Autodesk Inventor part; units mm, degrees
ref_plane "YZ Plane" through (0, 0, 0) normal (1, 0, 0) x (0, 1, 0)
ref_plane "XZ Plane" through (0, 0, 0) normal (0, 1, 0) x (-1, 0, 0)
ref_plane "XY Plane" through (0, 0, 0) normal (0, 0, 1) x (1, 0, 0)
sketch "Эскиз1" plane through (0, 0, 0) normal (0, 0, 1) x (1, 0, 0)
  line L0 (-74.5, -35) -> (74.5, -35)
  line L1 (74.5, -35) -> (74.5, 35)
  line L2 (74.5, 35) -> (-74.5, 35)
  line L3 (-74.5, 35) -> (-74.5, -35)
  line L4 (-74.5, -35) -> (74.5, 35) construction
  line L5 (74.5, -35) -> (-74.5, 35) construction
  point P0 (0, 0)
  dimension "d0" = 149
  dimension "d1" = 70
extrude "Выдавливание1" add sketch "Эскиз1" along normal blind 3
sketch "Эскиз2" plane through (0, 0, 3) normal (0, 0, 1) x (1, 0, 0)
  line L0 (74.5, -35) -> (74.5, 35)
  line L1 (74.5, 25) -> (71.5, 25)
  line L2 (71.5, 25) -> (71.5, 15)
  line L3 (71.5, 15) -> (74.5, 15)
  line L4 (74.5, 15) -> (74.5, 25)
  line L5 (74.5, 35) -> (-74.5, 35)
  point P0 (0, 0)
  dimension "d4" = 3
  dimension "d5" = 10
  dimension "d6" = 10
extrude "Выдавливание2" cut sketch "Эскиз2" against normal blind 3
pattern_linear "Прямоуг.массив1" count 3 spacing 20 along (0, -1, 0) of "Выдавливание2"
mirror "Зеркальное отражение1" about plane through (0, 0, 0) normal (1, 0, 0) of "Выдавливание2", "Прямоуг.массив1"
sketch "Эскиз3" plane through (0, 0, 3) normal (0, 0, 1) x (1, 0, 0)
  line L0 (-74.5, -35) -> (74.5, -35)
  line L1 (-50, -35) -> (50, -35)
  line L2 (50, -35) -> (50, -38)
  line L3 (50, -38) -> (-50, -38)
  line L4 (-50, -38) -> (-50, -35)
  line L5 (0, 0) -> (0, -8.2609)
  line L6 (-74.5, -25) -> (-74.5, -35)
  dimension "d12" = 3
  dimension "d13" = 24.5
extrude "Выдавливание3" add sketch "Эскиз3" against normal blind 3
sketch "Эскиз4" plane through (0, 0, 3) normal (0, 0, 1) x (1, 0, 0)
  line L0 (74.5, 35) -> (-74.5, 35)
  line L1 (-74.5, 35) -> (-64.5, 35)
  line L2 (-64.5, 35) -> (-64.5, 32)
  line L3 (-64.5, 32) -> (-74.5, 32)
  line L4 (-74.5, 32) -> (-74.5, 35)
  line L5 (-74.5, 35) -> (-74.5, 25)
  point P0 (0, 0)
  point P1 (-64.5, 35)
  dimension "d16" = 10
  dimension "d17" = 3
  dimension "d18" = 0
extrude "Выдавливание4" cut sketch "Эскиз4" against normal blind 3
pattern_linear "Прямоуг.массив2" count 8 spacing 20 along (1, 0, 0) of "Выдавливание4"
properties part number "000.104 - Back wall"
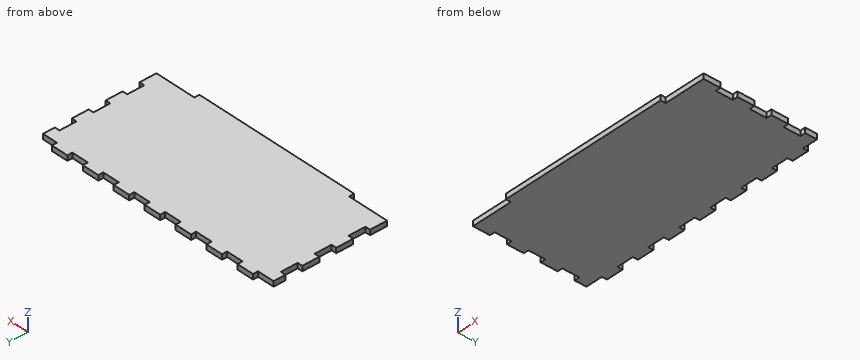
Work out the finished part from the listing and answer in its coordinate system (mm). Give positions to 0.01 mm unless a question says otherwise; leave off trailing zeros. Write each loop counter-clockwise with the first axis right and the second up, starting at its lowest first coordinate (ties: lowest second). Pieces come first, ordered by that corner, then holes.
(1) The part is cut by section A-A on y = 2. Write down the section's boundary in (x, z).
Final values:
outline: (-71.5, 0) - (71.5, 0) - (71.5, 3) - (-71.5, 3) - close
(2) Straight lines are drawn through the part: line 1 (Y direction, x = 12, z = 0.85); line 2 (X direction, y = -20, z = 1.55); line 3 (Y direction, x = 64.5, z = 1.75). For each, find the intervals that lie inside material, in ascending order.
Final values:
line 1: y = -38 to 32
line 2: x = -71.5 to 71.5
line 3: y = -35 to 35
(3) The part is cut by section B-B on x = -62.5. Write down the section's boundary in (y, z), plus the area to 3 significant figures.
Final values:
outline: (-35, 0) - (35, 0) - (35, 3) - (-35, 3) - close
area: 210 mm2
(4) Flat-ended cylindrical pins translate along their axes: pin 1 Ø1 at (y, z) = (-22, 1) entering from +X; pin 2 Ø1.5 at (x, z) = (-65, 2) entering from -Y; pin 3 Ø1.5 at (y, z) = (34, 2) entering from +X. Find the tip coordinate at first contact, or state that the pin passes through.
Final values:
pin 1: stops at x = 71.5
pin 2: stops at y = -35
pin 3: stops at x = 65.5
